```python
from build123d import *
from OCP.BRepFilletAPI import BRepFilletAPI_MakeChamfer

# Parameters (mm, degrees)
SKETCH11_W     = 6
SKETCH11_H     = 6
EXTRUDE8_DEPTH = 10
CHAMFER1_SIZE  = 1
CHAMFER2_SIZE  = 1
CHAMFER3_SIZE  = 1
CHAMFER3_SIZE2 = 1.732050808
CHAMFER4_SIZE  = 1
CHAMFER4_SIZE2 = 1.732050808


with BuildPart() as part:
    # Sketch11 → Extrude8 (new body)
    with BuildSketch(Plane(origin=(0, 0, 0), x_dir=(1, 0, 0), z_dir=(0, 1, 0))):
        Rectangle(SKETCH11_W, SKETCH11_H)
    extrude(amount=EXTRUDE8_DEPTH)

    # Chamfer1
    chamfer1_edges = [part.edges().sort_by_distance(p)[0] for p in [
        (3, 5, -3),
        (-3, 5, 3),
    ]]
    chamfer(chamfer1_edges, length=CHAMFER1_SIZE)

    # Chamfer2
    chamfer2_edges = [part.edges().sort_by_distance(p)[0] for p in [
        (-3, 5, -3),
        (3, 5, 3),
    ]]
    chamfer(chamfer2_edges, length=CHAMFER2_SIZE)

    # Chamfer3: one chamfer whose edges measure the first distance from different faces: ONE call of the kernel's chamfer builder (chamfer() names one face for all edges)
    chamfer3_edges_1 = [part.edges().sort_by_distance(p)[0] for p in [
        (0, 10, 3),
    ]]
    chamfer3_side_1 = [part.faces().sort_by_distance(p)[0] for p in [
        (0, 5, 3),
    ]]
    chamfer3_edges_2 = [part.edges().sort_by_distance(p)[0] for p in [
        (0, 10, -3),
    ]]
    chamfer3_side_2 = [part.faces().sort_by_distance(p)[0] for p in [
        (0, 5, -3),
    ]]
    chamfer3 = BRepFilletAPI_MakeChamfer(part.part.solid().wrapped)
    for e in chamfer3_edges_1:
        chamfer3.Add(CHAMFER3_SIZE, CHAMFER3_SIZE2, e.wrapped, chamfer3_side_1[0].wrapped)  # the first distance lies on this face
    for e in chamfer3_edges_2:
        chamfer3.Add(CHAMFER3_SIZE, CHAMFER3_SIZE2, e.wrapped, chamfer3_side_2[0].wrapped)  # the first distance lies on this face
    add(Compound.cast(chamfer3.Shape()), mode=Mode.REPLACE)

    # Chamfer4: one chamfer whose edges measure the first distance from different faces: ONE call of the kernel's chamfer builder (chamfer() names one face for all edges)
    chamfer4_edges_1 = [part.edges().sort_by_distance(p)[0] for p in [
        (3, 10, 0),
    ]]
    chamfer4_side_1 = [part.faces().sort_by_distance(p)[0] for p in [
        (3, 4.962121611, 0),
    ]]
    chamfer4_edges_2 = [part.edges().sort_by_distance(p)[0] for p in [
        (-3, 10, 0),
    ]]
    chamfer4_side_2 = [part.faces().sort_by_distance(p)[0] for p in [
        (-3, 4.962121611, 0),
    ]]
    chamfer4 = BRepFilletAPI_MakeChamfer(part.part.solid().wrapped)
    for e in chamfer4_edges_1:
        chamfer4.Add(CHAMFER4_SIZE, CHAMFER4_SIZE2, e.wrapped, chamfer4_side_1[0].wrapped)  # the first distance lies on this face
    for e in chamfer4_edges_2:
        chamfer4.Add(CHAMFER4_SIZE, CHAMFER4_SIZE2, e.wrapped, chamfer4_side_2[0].wrapped)  # the first distance lies on this face
    add(Compound.cast(chamfer4.Shape()), mode=Mode.REPLACE)


solid = part.part
```
Build history of the part. All positions in model axes, mm. Give positions to 0.01 mm unless a question says otherwise; leave off trailing zeros. Order: outer loops, then holes, each group sorted by start corner. A loop starts at its lowest first (then second) coordinate and runs counter-clockwise, first axis right, second up. Notation, with made-up numbers: M 23.25,-8 L 53.25,-8 A25 cw 53.25,23 Z; hole C 89.5,50.25 d6. An arc over 180 degrees is marked long. Write item = value, one per line. Start each with the question number.
(1) Slice it at C-C on z = 0.95. Write the cut outline in (x, y).
(2) Slice it at A-A on x = -0.1. Write the cut outline in (y, z).
(3) Slice it at B-B on y = 2.75. Write the cut outline in (x, z).
(4) Probe L1, parallel to X at y = 7.25, z = 2.35; L2, parallel to Y at x = -2.3, z = -1.1; L3, parallel to Y at x = -2.2, z = -0.2. List the from-to ranges inside material, lowest first. Write a range as [from, to].
Responses:
q1.outline = M -3,0 L 3,0 L 3,9 L 1.27,10 L -1.27,10 L -3,9 Z
q2.outline = M 0,-3 L 9,-3 L 10,-1.27 L 10,1.27 L 9,3 L 0,3 Z
q3.outline = M -3,-2 L -2,-3 L 2,-3 L 3,-2 L 3,2 L 2,3 L -2,3 L -3,2 Z
q4.L1 = [-2.65, 2.65]
q4.L2 = [0, 9.4]
q4.L3 = [0, 9.46]
